```python
from build123d import *

# Parameters (mm, degrees)
SKETCH1_R           = 1.6
BOSS_EXTRUDE1_DEPTH = 1
SKETCH5_W           = 2
SKETCH5_H           = 4.5
SKETCH5_H_2         = 4
CUT_EXTRUDE1_DEPTH  = 4
SKETCH4_W           = 21.2
SKETCH4_H           = 6
CUT_EXTRUDE2_DEPTH  = 4
SKETCH2_R           = 7.5
CUT_EXTRUDE3_DEPTH  = 4


with BuildPart() as part:
    # Sketch1 → Boss-Extrude1 (new body)
    with BuildSketch(Plane.XY):
        Polygon((20.734205703, -15.283501687), (20.734205703, -27.983501687), (-24.265794297, -27.983501687), (-24.265794297, -15.283501687), (-17.985794297, -15.283501687), (-17.985794297, -16.633501687), (-15.265794297, -16.633501687), (-15.265794297, -12.383501687), (-16.465794297, -12.383501687), (-16.465794297, -3.583501687), (-24.265794297, -3.583501687), (-24.265794297, 42.016498313), (20.734205703, 42.016498313), (20.734205703, -3.583501687), (12.934205703, -3.583501687), (12.934205703, -15.283501687), align=None)
        with Locations((-21.265794297, 39.016498313)):
            Circle(SKETCH1_R, mode=Mode.SUBTRACT)
        with Locations((17.734205703, 39.016498313)):
            Circle(SKETCH1_R, mode=Mode.SUBTRACT)
        with Locations((-21.265794297, -24.983501687)):
            Circle(SKETCH1_R, mode=Mode.SUBTRACT)
        with Locations((17.734205703, -24.983501687)):
            Circle(SKETCH1_R, mode=Mode.SUBTRACT)
    extrude(amount=BOSS_EXTRUDE1_DEPTH)

    # Sketch5 → Cut-Extrude1 (cut)
    with BuildSketch(Plane.XY.offset(1)):
        with Locations((-17.515794297, -1.733501687)):
            Rectangle(SKETCH5_W, SKETCH5_H)
        with Locations((3.734205703, -4.383501687)):
            Rectangle(SKETCH5_W, SKETCH5_H_2)
    extrude(amount=-CUT_EXTRUDE1_DEPTH, mode=Mode.SUBTRACT)

    # Sketch4 → Cut-Extrude2 (cut)
    with BuildSketch(Plane.XY.offset(1)):
        with Locations((-1.765794297, -21.483501687)):
            Rectangle(SKETCH4_W, SKETCH4_H)
        with Locations((-1.765794297, 34.616498313)):
            Rectangle(SKETCH4_W, SKETCH4_H)
    extrude(amount=-CUT_EXTRUDE2_DEPTH, mode=Mode.SUBTRACT)

    # Sketch2 → Cut-Extrude3 (cut)
    with BuildSketch(Plane.XY.offset(1)):
        with Locations((-11.365794297, 7.016498313)):
            Circle(SKETCH2_R)
        with Locations((7.734205703, 7.016498313)):
            Circle(SKETCH2_R)
    extrude(amount=-CUT_EXTRUDE3_DEPTH, mode=Mode.SUBTRACT)


solid = part.part
```
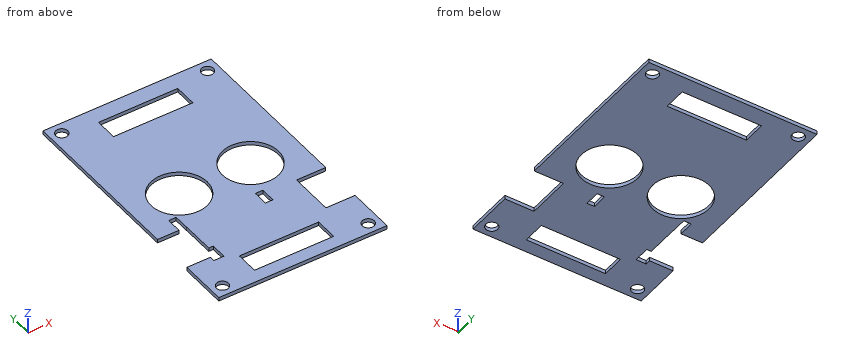
Model file for the job. Use its own axes, mm. Give positions to 0.01 mm unless a question says otherwise; leave off trailing zeros. Order: outer loops, then holes, each group sorted by start corner. A loop starts at its lowest first (then second) coordinate and runs counter-clockwise, first axis right, second up.
1) Saw through at C-C, the plane z = 0.45. Count the separate pieces of the cut face and the enclosed holes in it, then the cut area to 3 significant figures.
2) Saw through at B-B, the plane x = -5. Write the cut outline in (y, z).
3) Wall check: probe 1 along Y at (x, z) = (-3, 0.5); probe 2 along X at (y, z) = (35, 0.1); probe 3 along Y at (x, z) = (-5, 0.85). Give the ranges that are in metal, low to high.
4) Saw through at D-D, the plane x = 1.5. Write the cut outline in (y, z), then the cut area to 3 significant figures.
5) Saw through at A-A, the plane y = 11. Write the cut outline in (x, z).
Computed:
1. separate pieces: 1
1. enclosed holes: 9
1. area: 2,300 mm2
2. outline: (-27.98, 0) - (-24.48, 0) - (-24.48, 1) - (-27.98, 1) - close; (-18.48, 0) - (3.05, 0) - (3.05, 1) - (-18.48, 1) - close; (10.98, 0) - (31.62, 0) - (31.62, 1) - (10.98, 1) - close; (37.62, 0) - (42.02, 0) - (42.02, 1) - (37.62, 1) - close
3. probe 1: y = -27.98 to -24.48, -18.48 to 31.62, 37.62 to 42.02
3. probe 2: x = -24.27 to -12.37, 8.83 to 20.73
3. probe 3: y = -27.98 to -24.48, -18.48 to 3.05, 10.98 to 31.62, 37.62 to 42.02
4. outline: (-27.98, 0) - (-24.48, 0) - (-24.48, 1) - (-27.98, 1) - close; (-18.48, 0) - (2.85, 0) - (2.85, 1) - (-18.48, 1) - close; (11.19, 0) - (31.62, 0) - (31.62, 1) - (11.19, 1) - close; (37.62, 0) - (42.02, 0) - (42.02, 1) - (37.62, 1) - close
4. area: 49.7 mm2
5. outline: (-24.27, 0) - (-17.72, 0) - (-17.72, 1) - (-24.27, 1) - close; (-5.01, 0) - (1.38, 0) - (1.38, 1) - (-5.01, 1) - close; (14.09, 0) - (20.73, 0) - (20.73, 1) - (14.09, 1) - close
